```python
from build123d import *

# Parameters (mm, degrees)
EXTRU_MINCE1_DEPTH      = 128
ESQUISSE2_R             = 2.5
ENL_V_MAT_EXTRU_1_DEPTH = 10
ESQUISSE3_R             = 2.5
ESQUISSE3_W             = 18
ESQUISSE3_H             = 18.5
ENL_V_MAT_EXTRU_2_DEPTH = 10
ESQUISSE4_R             = 1.5
ENL_V_MAT_EXTRU_3_DEPTH = 5
ESQUISSE5_R             = 1.5
ENL_V_MAT_EXTRU_4_DEPTH = 5


with BuildPart() as part:
    # Esquisse1 → Extru.-Mince1 (new, symmetric)
    with BuildSketch(Plane(origin=(0, 0, 0), x_dir=(0, 0, -1), z_dir=(1, 0, 0))):
        Polygon((-20, 0), (0, 0), (0, -20), (-1.5, -20), (-1.5, -1.5), (-20, -1.5), align=None)
    extrude(amount=EXTRU_MINCE1_DEPTH, both=True)

    # Esquisse2 → Enlèv. mat.-Extru.1 (cut)
    with BuildSketch(Plane.XY.offset(1.5)):
        with Locations((-120, -10)):
            Circle(ESQUISSE2_R)
        with Locations(Location((120, -10, 0), (0, 0, 90))):
            Circle(ESQUISSE2_R)
    extrude(amount=-ENL_V_MAT_EXTRU_1_DEPTH, mode=Mode.SUBTRACT)

    # Esquisse3 → Enlèv. mat.-Extru.2 (cut)
    with BuildSketch(Plane.XZ.offset(1.5)):
        with Locations(Location((-38, 11.5, 0), (0, 0, 270))):
            Circle(ESQUISSE3_R)
        with Locations(Location((38, 11.5, 0), (0, 0, 90))):
            Circle(ESQUISSE3_R)
        with Locations((-119, 10.75)):
            Rectangle(ESQUISSE3_W, ESQUISSE3_H)
        with Locations((119, 10.75)):
            Rectangle(ESQUISSE3_W, ESQUISSE3_H)
    extrude(amount=-ENL_V_MAT_EXTRU_2_DEPTH, mode=Mode.SUBTRACT)

    # Esquisse4 → Enlèv. mat.-Extru.3 (cut)
    with BuildSketch(Plane(origin=(0, 0, 0), x_dir=(1, 0, 0), z_dir=(0, 1, 0))):
        with Locations(Location((0, -10, 0), (0, 0, 270))):
            Circle(ESQUISSE4_R)
    extrude(amount=-ENL_V_MAT_EXTRU_3_DEPTH, mode=Mode.SUBTRACT)

    # Esquisse5 → Enlèv. mat.-Extru.4 (cut)
    with BuildSketch(Plane(origin=(0, 0, 0), x_dir=(-1, 0, 0), z_dir=(0, 0, -1))):
        with Locations(Location((-20, -10, 0), (0, 0, 90))):
            Circle(ESQUISSE5_R)
        with Locations(Location((20, -10, 0), (0, 0, 90))):
            Circle(ESQUISSE5_R)
    extrude(amount=-ENL_V_MAT_EXTRU_4_DEPTH, mode=Mode.SUBTRACT)


solid = part.part
```
For this review, take the finished solid that the model builds, in its own axes (mm). A direction names the side the tool comes from. Round coordinates to 2 decimals unless told otherwise and drop trailing zeros. Write each loop counter-clockwise with the first axis right and the second up, starting at its lowest first coordinate (ties: lowest second). Pieces come first, ordered by that corner, then holes. Notation, with made-up numbers: (-40, -17.5) - (16, -17.5) arc R13 cw to (16, -2.5) - close; hole circle Ø5 at (-18.5, 16.5). An arc over 180 degrees is marked (long way). Write each question's results on one line, items separated by ' | '.
Item 1: Take a section at A-A on x = -38. State the section outline as (y, z) points.
Calculated:
outline: (-20, 0) - (0, 0) - (0, 9) - (-1.5, 9) - (-1.5, 1.5) - (-20, 1.5) - close; (-1.5, 14) - (0, 14) - (0, 20) - (-1.5, 20) - close
Item 2: For faces 3 (the face through (2, -1.5, 11)), 4 (the face through (2, 0, 10)), list the 3-axis set-ups (+Z, -Z, +X, -X, +Y, -Y) from which the entire face can be reached by the end or side of a thin tool; tool diameter is ignored.
Calculated:
face 3: +Z, +X, -X, -Y | face 4: +Z, -Z, +X, -X, +Y
Item 3: Take a section at D-D on y = -5. State the section outline as (x, z) points, then the cut area to 3 significant figures.
Calculated:
outline: (-128, 0) - (128, 0) - (128, 1.5) - (-128, 1.5) - close | area: 384 mm^2
Item 4: To check wall thickness, follow line 1 along Y through (x, z) = (65, 11.75); line 2 along Z through (x, y) = (-14, -3.25); line 3 along X through (y, z) = (-0.6, 10). State the ranges of each line that lie inside material, in increasing order. Write a range as from..to.
Calculated:
line 1: y = -1.5..0 | line 2: z = 0..1.5 | line 3: x = -110..-40, -36..-1.5, 1.5..36, 40..110
Item 5: Take a section at B-B on x = -120. State the section outline as (y, z) points.
Calculated:
outline: (-20, 0) - (-12.5, 0) - (-12.5, 1.5) - (-20, 1.5) - close; (-7.5, 0) - (0, 0) - (0, 1.5) - (-7.5, 1.5) - close
Item 6: Take a section at C-C on z = 16.5. State the section outline as (x, y) points.
Calculated:
outline: (-110, -1.5) - (110, -1.5) - (110, 0) - (-110, 0) - close
Item 7: Draft analysis for pull direction X (two halves, no side actions). For faces 1 (the face through (2, -10, 0)), 2 (the face through (40.44, -0.76, 10.96)), state which applies: pulls with the +X half, pulls with the -X half, needs draft (parallel to the pull), parting line crosses it, or undercut.
Calculated:
face 1: needs draft | face 2: undercut
Item 8: For pin 1 (4 mm diameter, centred on x = -31.5, y = -16, fed in from +Z); pin 2 (8 mm diameter, centred on x = -38, z = 11.5, fed in from -Y); pin 3 (0.8 mm diameter, centred on y = -0.5, z = 12, fed in from +X), all flat-tipped, find the tip position at first contact; note any pin that passes through.
Calculated:
pin 1: stops at z = 1.5 | pin 2: stops at y = -1.5 | pin 3: stops at x = 110
